Design review of the part built by this model. Coordinates are the model's own, in mm. Face numbers are marked on the shaded views. A direction names the side the tool comes from. Coordinates: 2 decimals unless noted, no trailing zeros. Write each loop counter-clockwise with the first axis right and the second up, starting at its lowest first coordinate (ties: lowest second). Pieces come first, ordered by that corner, then holes. Notation, with made-up numbers: (71.5, 87.5) - (85.5, 87.5) arc R20 cw to (85.5, 99.5) - close; hole circle Ø1 at (41.25, 23). An arc over 180 degrees is marked (long way). Use a Markdown table: item, result.
from build123d import *

# Parameters (mm, degrees)
SKETCH1_R           = 0.75
BOSS_EXTRUDE1_DEPTH = 1.5
SKETCH2_W           = 3.2
SKETCH2_H           = 4.8
BOSS_EXTRUDE2_DEPTH = 1


with BuildPart() as part:
    # Sketch1 → Boss-Extrude1 (new body)
    with BuildSketch(Plane(origin=(0, 0, 0), x_dir=(1, 0, 0), z_dir=(0, 1, 0))):
        with BuildLine():
            Line((-1.6, 9), (-1.6, 0))
            ThreePointArc((-1.6, 0), (0, -1.6), (1.6, 0))
            Line((1.6, 0), (1.6, 9))
            ThreePointArc((1.6, 9), (0, 10.6), (-1.6, 9))
        make_face()
        with Locations(Location((0, 9, 0), (0, 0, 270))):
            Circle(SKETCH1_R, mode=Mode.SUBTRACT)
        with Locations(Location((0, 0, 0), (0, 0, 270))):
            Circle(SKETCH1_R, mode=Mode.SUBTRACT)
    extrude(amount=BOSS_EXTRUDE1_DEPTH)

    # Sketch2 → Boss-Extrude2 (add)
    with BuildSketch(Plane(origin=(0, 1.5, 0), x_dir=(1, 0, 0), z_dir=(0, 1, 0))):
        with Locations((0, 4.5)):
            Rectangle(SKETCH2_W, SKETCH2_H)
    extrude(amount=BOSS_EXTRUDE2_DEPTH)


solid = part.part
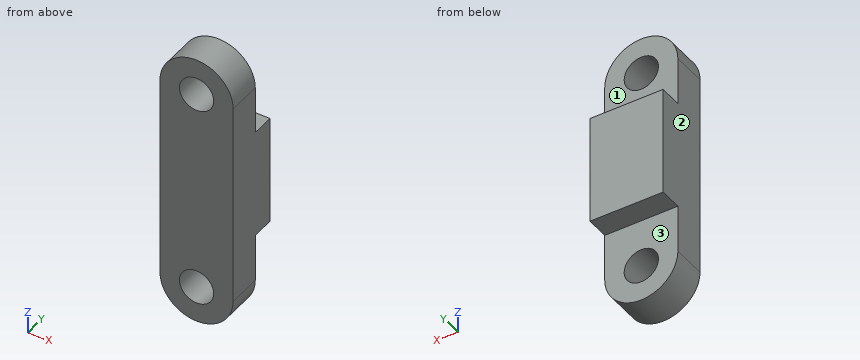
(1) For L1, parallel to Z at x = 0.2, y = 1.4; L2, parallel to Y at x = -1.4, z = -1.5; L3, parallel to Z at x = 0.9, y = 1.75, list the stretches that pass through material, from the lowest coordinate up. Write a range as from..to.
Determined:
| item | result |
|---|---|
| L1 | -10.59..-9.72, -8.28..-0.72, 0.72..1.59 |
| L2 | 0..1.5 |
| L3 | -6.9..-2.1 |
(2) Take a section at C-C on y = 0.35. Write out the cut boundary in (x, z).
Determined:
| item | result |
|---|---|
| outline | (-1.6, -9) arc R1.6 ccw to (1.6, -9) - (1.6, 0) arc R1.6 ccw to (-1.6, 0) - close; hole circle Ø1.5 at (0, -9); hole circle Ø1.5 at (0, 0) |
(3) Take a section at D-D on x = 1.25. Write out the cut boundary in (y, z).
Determined:
| item | result |
|---|---|
| outline | (0, -10) - (1.5, -10) - (1.5, -6.9) - (2.5, -6.9) - (2.5, -2.1) - (1.5, -2.1) - (1.5, 1) - (0, 1) - close |
(4) Take a section at A-A on x = 0. Write out the cut boundary in (y, z), and give its area (3 significant figures).
Determined:
| item | result |
|---|---|
| outline | (0, -10.6) - (1.5, -10.6) - (1.5, -9.75) - (0, -9.75) - close; (0, -8.25) - (1.5, -8.25) - (1.5, -6.9) - (2.5, -6.9) - (2.5, -2.1) - (1.5, -2.1) - (1.5, -0.75) - (0, -0.75) - close; (0, 0.75) - (1.5, 0.75) - (1.5, 1.6) - (0, 1.6) - close |
| area | 18.6 mm2 |
(5) Machinability: for the marked faces 1, 2 and 3, which of the approach directions +Z, -Z, +X, -X, +Y, -Y give a long, thin tool a straight path to every point of the face, cutting with its end or side? Answer none if there is none.
Determined:
| item | result |
|---|---|
| face 1 | +Z, +X, -X, +Y |
| face 2 | +Z, -Z, -X, +Y, -Y |
| face 3 | -Z, +X, -X, +Y |
(6) Take a section at B-B on z = -8.5. Write out the cut boundary in (x, y).
Determined:
| item | result |
|---|---|
| outline | (-1.6, 0) - (-0.56, 0) - (-0.56, 1.5) - (-1.6, 1.5) - close; (0.56, 0) - (1.6, 0) - (1.6, 1.5) - (0.56, 1.5) - close |
(7) For pin 1 (1.6 mm diameter, centred on x = -0.5, z = -8, fed in from +Y), flat-tipped, find the tip position at first contact; note if it passes through.
Determined:
| item | result |
|---|---|
| pin 1 | y = 1.5 |
